```python
from build123d import *

# Parameters (mm, degrees)
BOSS_EXTRUDE1_DEPTH = 0.508
SKETCH2_R           = 2.2479
CUT_EXTRUDE1_DEPTH  = 11.636172283
FILLET1_RADIUS      = 4.6228
FILLET1_LENGTH      = 1.016


with BuildPart() as part:
    # Sketch1 → Boss-Extrude1 (new, symmetric)
    with BuildSketch(Plane.XY):
        Polygon((-4.6228, 6.35), (4.6228, 6.35), (4.6228, -6.35), (2.1717, -6.35), (2.1717, -9.525), (-2.1717, -9.525), (-2.1717, -6.35), (-4.6228, -6.35), align=None)
    extrude(amount=BOSS_EXTRUDE1_DEPTH, both=True)

    # Sketch2 → Cut-Extrude1 (cut, through all)
    with BuildSketch(Plane.XY.offset(0.508)):
        with Locations((0, 1.8161)):
            Circle(SKETCH2_R)
    extrude(amount=-CUT_EXTRUDE1_DEPTH, mode=Mode.SUBTRACT)

    # Fillet1: full round fillet: the end face becomes a half cylinder, R = half its width
    fillet1_face = Plane((0, 6.35, 0), x_dir=(0, 0, 1), z_dir=(0, 1, 0))  # on the end face: x along it, z out of the body
    fillet1_slab = fillet1_face.offset(-FILLET1_RADIUS / 2) * Box(FILLET1_LENGTH, 2 * FILLET1_RADIUS, FILLET1_RADIUS, mode=Mode.PRIVATE)  # the body's end, R deep
    fillet1_round = Plane((0, 1.7272, 0), x_dir=(0, 1, 0), z_dir=(0, 0, 1)) * Cylinder(FILLET1_RADIUS, FILLET1_LENGTH, mode=Mode.PRIVATE)  # its axis R under the face
    add(fillet1_slab - fillet1_round, mode=Mode.SUBTRACT)


solid = part.part
```
Could you check a few things on this model? Use its own coordinates, in mm. A direction names the side the tool comes from. Give positions to 0.01 mm unless a question says otherwise; leave off trailing zeros. Loops run counter-clockwise (first coordinate to the right, second up) from the corner with the lowest first, then second, coordinate; pieces in that order, holes last. Notation, with made-up numbers: (36.25, 13) - (69.25, 13) arc R30 cw to (69.25, 51) - close; hole circle Ø3 at (-1.5, -16.5). An arc over 180 degrees is marked (long way). Answer in a Markdown table with one row per item. Add a question column.
Q1. Please list where these lines run through material, in increasing order: L1, parallel to Y at x = 0, z = -0.1 (3 decimals); L2, parallel to X at y = -6.75, z = 0.45; L3, parallel to Y at x = -1.75, z = 0 (3 decimals). Write a range as from..to.
Q2. If we section it at B-B (y = 1.5): List the corners of the cut face in (x, z) for me.
Q3. We'd pull the mould along X, two halves only. Please class faces 4 (the face through (-0.487, -0.378, 0.007)), 5 (the face through (2.172, -8, 0)), 6 (the face through (0, -1, 0.508)): +X half, -X half, draft (parallel to the pull), parting line (faces both ways), or undercut.
Q4. Which directions (+Z, -Z, +X, -X, +Y, -Y) give clear straight access to the entire face, cutting with the end or side of a thin tool? Please do faces 1 (the face through (-4.623, -2, 0)), 2 (the face through (-3, -6.35, 0)), 3 (the face through (3, -6.35, 0)).
Q5. If we section it at D-D (y = -8.5): List the corners of the cut face in (x, z) for me.
Q6. For pin 1 (0.5 mm diameter, centred on y = -7.5, z = 0, fed in from -X), with a flat end and sliding along its axis, tell me the tip position at first contact or that it passes through.
Q7. If we section it at A-A (x = 0): List the corners of the cut face in (y, z) for me (3 decimals), plus the area to 3 significant figures.
Q8. If we section it at C-C (z = 0.1): List the corners of the cut face in (x, y) for me (3 decimals).
The answers:
| question | item | result |
|---|---|---|
| 1 | L1 | y = -9.525..-0.432, 4.064..6.35 |
| 1 | L2 | x = -2.17..2.17 |
| 1 | L3 | y = -9.525..0.405, 3.227..6.006 |
| 2 | outline | (-4.62, -0.51) - (-2.23, -0.51) - (-2.23, 0.51) - (-4.62, 0.51) - close; (2.23, -0.51) - (4.62, -0.51) - (4.62, 0.51) - (2.23, 0.51) - close |
| 3 | face 4 | undercut |
| 3 | face 5 | +X half |
| 3 | face 6 | draft |
| 4 | face 1 | +Z, -Z, -X, +Y, -Y |
| 4 | face 2 | +Z, -Z, -X, -Y |
| 4 | face 3 | +Z, -Z, +X, -Y |
| 5 | outline | (-2.17, -0.51) - (2.17, -0.51) - (2.17, 0.51) - (-2.17, 0.51) - close |
| 6 | pin 1 | stops at x = -2.17 |
| 7 | outline | (-9.525, -0.508) - (-0.432, -0.508) - (-0.432, 0.508) - (-9.525, 0.508) - close; (4.064, -0.508) - (6.35, -0.508) - (6.35, 0.508) - (4.064, 0.508) - close |
| 7 | area | 11.6 mm^2 |
| 8 | outline | (-4.623, -6.35) - (-2.172, -6.35) - (-2.172, -9.525) - (2.172, -9.525) - (2.172, -6.35) - (4.623, -6.35) - (4.623, 1.727) arc R4.623 ccw to (-4.623, 1.727) - close; hole circle Ø4.496 at (0, 1.816) |
